Geometry: see drawing. Coordinates: mm, zero at the bounding-box minimum. Round coordinates to 2 decimals unless told otherwise and drop trailing zeros. Loops run counter-clockwise (first coordinate to the right, second up) from the corner with the lowest first, then second, coordinate; pieces in that order, holes last. Notation, with made-up numbers: (5, 10.25) - (33, 10.25) arc R28 cw to (33, 47.25) - close; hole circle Ø11 at (57.5, -31.5). An arc over 180 degrees is marked (long way). Return JSON: item names as keys, results as strings. Group by question number.
1. Section A-A on x = 71.12. Return loops of the section in (y, z).
2. First-contact query: pin 1 Ø6.5 at (x, y) = (71.12, 5) entering from +Z; pin 2 Ø0.5 at (y, z) = (45.5, 0.5) entering from +X; pin 3 Ø0.8 at (x, z) = (128, 0.5) entering from +Y (1 decimal); pin 4 Ø0.5 at (y, z) = (45, 0.5) entering from -X. Flat tips, straight axial feed; report the tip coordinate or a pass-through.
3. Section C-C on z = 0.6. Return loops of the section in (x, y) (1 decimal).
4. Material intervals for probe 1 along Y at (x, z) = (71.12, 1); probe 2 along Y at (x, z) = (42, 0.9) (1 decimal); probe 3 along X at (y, z) = (7, 0.25) (1 decimal), sorted ascending.
5. Section B-B on y = 5. Return loops of the section in (x, z), and give its area (3 significant figures).
6. Section D-D on x = 120.5. Return loops of the section in (y, z) (1 decimal).
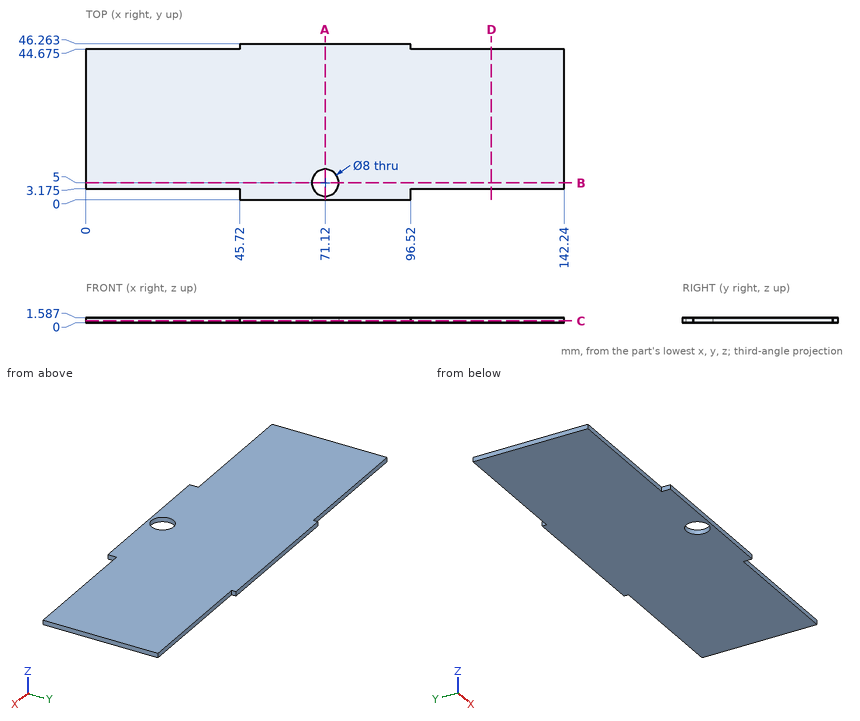
Taken from the geometry:
{
 "1": {"outline": "(0, 0) - (1, 0) - (1, 1.59) - (0, 1.59) - close; (9, 0) - (46.26, 0) - (46.26, 1.59) - (9, 1.59) - close"},
 "2": {"pin 1": "through", "pin 2": "x = 96.52", "pin 3": "y = 44.7", "pin 4": "x = 45.72"},
 "3": {"outline": "(0, 3.2) - (45.7, 3.2) - (45.7, 0) - (96.5, 0) - (96.5, 3.2) - (142.2, 3.2) - (142.2, 44.7) - (96.5, 44.7) - (96.5, 46.3) - (45.7, 46.3) - (45.7, 44.7) - (0, 44.7) - close; hole circle Ø8 at (71.1, 5)"},
 "4": {"probe 1": "0 to 1, 9 to 46.26", "probe 2": "3.2 to 44.7", "probe 3": "0 to 67.7, 74.6 to 142.2"},
 "5": {"outline": "(0, 0) - (67.12, 0) - (67.12, 1.59) - (0, 1.59) - close; (75.12, 0) - (142.24, 0) - (142.24, 1.59) - (75.12, 1.59) - close", "area": "213 mm2"},
 "6": {"outline": "(3.2, 0) - (44.7, 0) - (44.7, 1.6) - (3.2, 1.6) - close"}
}
